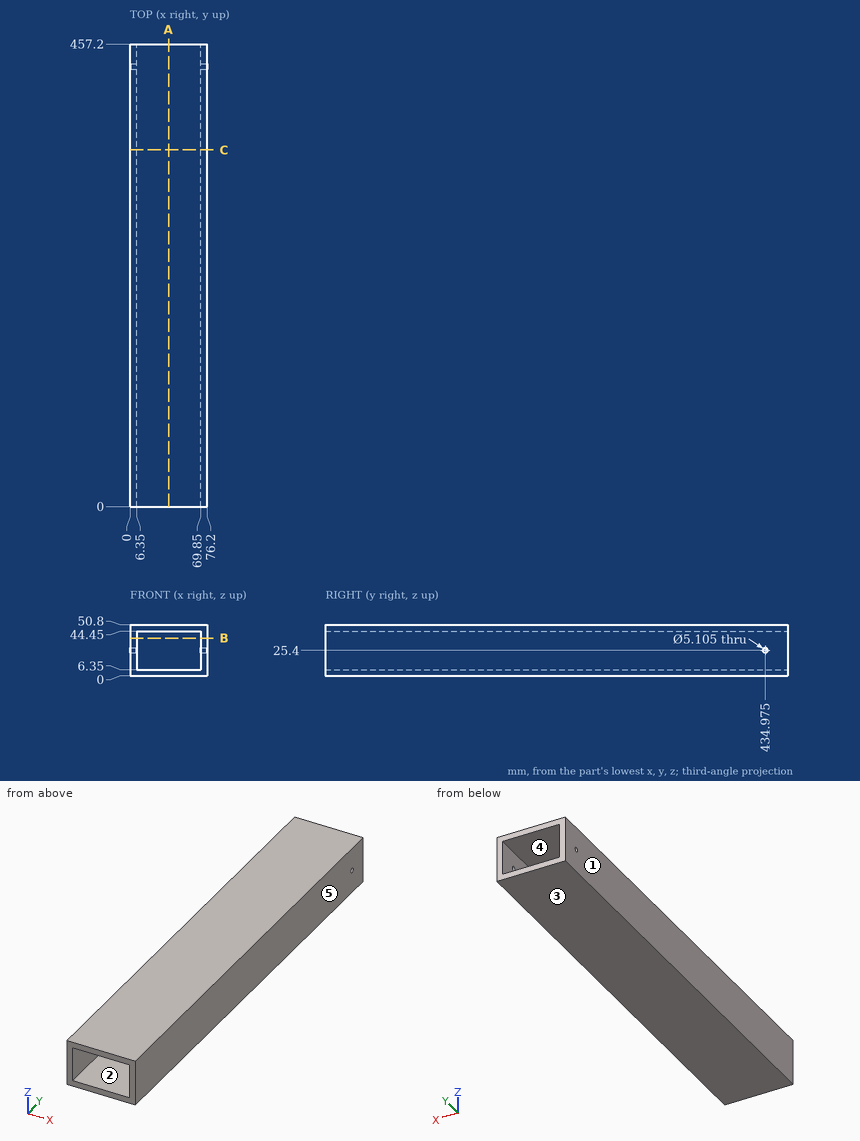
Design review of the part shown in the three views and the two pictorial views. Dimensions are in mm from the part's minimum x, y and z. A direction names the side the tool comes from. Round coordinates to 2 decimals unless told otherwise and drop trailing zeros. Loops run counter-clockwise (first coordinate to the right, second up) from the corner with the lowest first, then second, coordinate; pieces in that order, holes last. Notation, with made-up numbers: (-33, 34) -> (-16, 34) arc R18 cw to (-16, 60) -> close; hole circle Ø6 at (38, 71). An arc over 180 degrees is marked (long way). Answer as a JSON object with one key per item and string values. Group by question number.
1) For the marked faces 4 and 5, list the 3-axis set-ups (+Z, -Z, +X, -X, +Y, -Y) from which the entire face can be reached by the end or side of a thin tool; tool diameter is ignored.
2) We need section A-A on x = 38. Write out the cut boundary in (y, z).
3) We need section B-B on z = 37.5. Write out the cut boundary in (x, y).
4) We need section C-C on y = 352.5. Write out the cut boundary in (x, z), then the cut area to 3 significant figures.
5) For line 1 (Y direction, x = 3, z = 25); line 2 (Z direction, x = 61, y = 106.5); line 3 (X direction, y = 245, z = 38), list the stretches that pass through material, from the lowest coordinate up. Write a range as [from, to].
6) For pin 1 Ø1.5 at (x, z) = (27.5, 7.5) entering from +Y, flat-tipped, find the tip position at first contact; note if it passes through.
7) Mouldability with a two-part tool opening along Z and no side actions: class the marked faces 1, 2 and 3 as released by +Z, released by -Z, zero draft, split by the parting line, or undercut.
Result set:
{
 "1": {"face 4": "+Y, -Y", "face 5": "+Z, -Z, +X, +Y, -Y"},
 "2": {"outline": "(0, 0) -> (457.2, 0) -> (457.2, 6.35) -> (0, 6.35) -> close; (0, 44.45) -> (457.2, 44.45) -> (457.2, 50.8) -> (0, 50.8) -> close"},
 "3": {"outline": "(0, 0) -> (6.35, 0) -> (6.35, 457.2) -> (0, 457.2) -> close; (69.85, 0) -> (76.2, 0) -> (76.2, 457.2) -> (69.85, 457.2) -> close"},
 "4": {"outline": "(0, 0) -> (76.2, 0) -> (76.2, 50.8) -> (0, 50.8) -> close; hole (6.35, 6.35) -> (69.85, 6.35) -> (69.85, 44.45) -> (6.35, 44.45) -> close", "area": "1,450 mm²"},
 "5": {"line 1": "[0, 432.45], [437.5, 457.2]", "line 2": "[0, 6.35], [44.45, 50.8]", "line 3": "[0, 6.35], [69.85, 76.2]"},
 "6": {"pin 1": "through"},
 "7": {"face 1": "zero draft", "face 2": "undercut", "face 3": "released by -Z"}
}
